from build123d import *

# Parameters (mm, degrees)
F1_DEPTH = 3


with BuildPart() as f1:
    # F0 (on Top) → F1 (new body)
    with BuildSketch(Plane.XY):
        with BuildLine():
            Line((16.723475, 5.431714), (8.751905, 14.74098))
            Line((8.751905, 14.74098), (4.802136, 11.358773))
            Line((4.802136, 11.358773), (-4.802136, 11.358773))
            Line((-4.802136, 11.358773), (-8.751905, 14.740979))
            Line((-8.751905, 14.740979), (-16.723475, 5.431713))
            Line((-16.723475, 5.431713), (-16.723475, 0))
            Line((-16.723475, 0), (-16.723475, -5.431713))
            Line((-16.723475, -5.431713), (-8.751905, -14.740979))
            Line((-8.751905, -14.740979), (-3.890651, -10.578264))
            Line((-3.890651, -10.578264), (-9.43802, -4.1))
            Line((-9.43802, -4.1), (-8.712763, -4.1))
            Line((-8.712763, -4.1), (-5.826839, -5.033681))
            ThreePointArc((-5.826839, -5.033681), (-4.72977, -6.076123), (-3.45, -6.883858))
            Line((-3.45, -6.883858), (-3.45, -14.2))
            Line((-3.45, -14.2), (3.45, -14.2))
            Line((3.45, -14.2), (3.45, -6.883857))
            ThreePointArc((3.45, -6.883857), (4.72977, -6.076123), (5.826838, -5.033681))
            Line((5.826838, -5.033681), (8.712763, -4.099999))
            Line((8.712763, -4.099999), (9.43802, -4.099999))
            Line((9.43802, -4.099999), (3.890651, -10.578264))
            Line((3.890651, -10.578264), (8.751905, -14.74098))
            Line((8.751905, -14.74098), (16.723475, -5.431714))
            Line((16.723475, -5.431714), (16.723475, 0))
            Line((16.723475, 0), (16.723475, 5.431714))
        make_face()
        with BuildLine():
            ThreePointArc((-2.25, -6.098155), (-3.833093, -5.249514), (-5.123475, -4))
            Line((-5.123475, -4), (-8.523475, -2.9))
            Line((-8.523475, -2.9), (-10.323475, -2.9))
            Line((-10.323475, -2.9), (-10.323475, -4))
            Line((-10.323475, -4), (-10.723475, -4))
            Line((-10.723475, -4), (-10.723475, -4.443783))
            Line((-10.723475, -4.443783), (-5.582645, -10.447288))
            Line((-5.582645, -10.447288), (-8.620929, -13.048985))
            Line((-8.620929, -13.048985), (-15.523475, -4.988134))
            Line((-15.523475, -4.988134), (-15.523475, 0))
            Line((-15.523475, 0), (-15.523475, 4.988134))
            Line((-15.523475, 4.988134), (-8.620929, 13.048985))
            Line((-8.620929, 13.048985), (-5.582645, 10.447288))
            Line((-5.582645, 10.447288), (-10.723475, 4.443783))
            Line((-10.723475, 4.443783), (-10.723475, 4))
            Line((-10.723475, 4), (-10.323475, 4))
            Line((-10.323475, 4), (-10.323475, 2.9))
            Line((-10.323475, 2.9), (-8.523475, 2.9))
            Line((-8.523475, 2.9), (-5.123475, 4))
            ThreePointArc((-5.123475, 4), (-3.028916, 5.751145), (-0.4, 6.487681))
            Line((-0.4, 6.487681), (-0.4, 7.3))
            Line((-0.4, 7.3), (0, 7.3))
            Line((0, 7.3), (0.4, 7.3))
            Line((0.4, 7.3), (0.4, 6.487681))
            ThreePointArc((0.4, 6.487681), (3.028916, 5.751145), (5.123475, 4))
            Line((5.123475, 4), (8.523475, 2.9))
            Line((8.523475, 2.9), (10.323475, 2.9))
            Line((10.323475, 2.9), (10.323475, 4))
            Line((10.323475, 4), (10.723475, 4))
            Line((10.723475, 4), (10.723475, 4.443783))
            Line((10.723475, 4.443783), (5.582645, 10.447288))
            Line((5.582645, 10.447288), (8.620929, 13.048985))
            Line((8.620929, 13.048985), (15.523475, 4.988134))
            Line((15.523475, 4.988134), (15.523475, 0))
            Line((15.523475, 0), (15.523475, -4.988134))
            Line((15.523475, -4.988134), (8.620929, -13.048985))
            Line((8.620929, -13.048985), (5.582645, -10.447288))
            Line((5.582645, -10.447288), (10.723475, -4.443783))
            Line((10.723475, -4.443783), (10.723475, -4))
            Line((10.723475, -4), (10.323475, -4))
            Line((10.323475, -4), (10.323475, -2.9))
            Line((10.323475, -2.9), (8.523475, -2.9))
            Line((8.523475, -2.9), (5.123475, -4))
            ThreePointArc((5.123475, -4), (3.833093, -5.249514), (2.25, -6.098155))
            Line((2.25, -6.098155), (2.25, -13))
            Line((2.25, -13), (-2.25, -13))
            Line((-2.25, -13), (-2.25, -6.098155))
        make_face(mode=Mode.SUBTRACT)
    extrude(amount=F1_DEPTH)


solid = f1.part
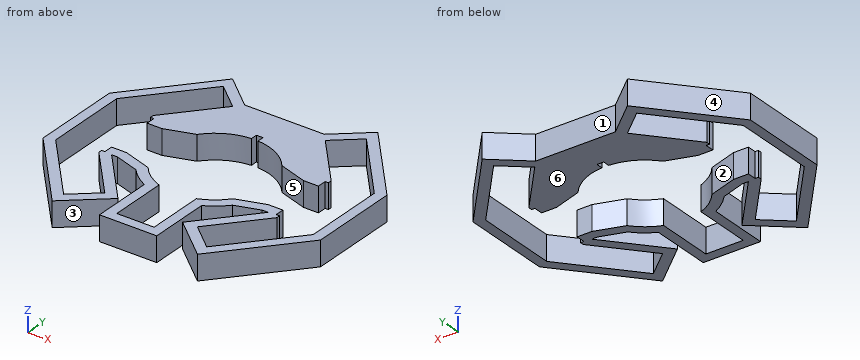
Input: part model. Units: mm. Frame: model coordinates. Face numbers are marked on the shaded views. A direction names the side the tool comes from. Coordinates: 2 decimals unless noted, no trailing zeros. Order: outer loops, then holes, each group sorted by start corner. A loop starts at its lowest first (then second) coordinate and runs counter-clockwise, first axis right, second up.
1. Contact query for flat-ended pins moving along their axis: P1, Ø1.4, axis at x = 9.5, z = 1, coming from the +Y side; P2, Ø1.5, axis at x = 0.5, z = 1, coming from the +Y side; P3, Ø1, axis at y = 7.5, z = 1.5, coming from the -X side. Output: stop coordinate, or through.
Checked values:
P1: stops at y = 14.68
P2: stops at y = 11.36
P3: stops at x = -15.38
2. Cut plane C-C, the plane y = 0.5. Return loops of the section in (x, z), plus the area to 3 significant figures.
Checked values:
outline: (-16.72, 0) - (-15.52, 0) - (-15.52, 3) - (-16.72, 3) - close; (15.52, 0) - (16.72, 0) - (16.72, 3) - (15.52, 3) - close
area: 7.20 mm2
3. Cut plane D-D, the plane y = -11. Return loops of the section in (x, z), plus the area to 3 significant figures.
Checked values:
outline: (-11.96, 0) - (-10.38, 0) - (-10.38, 3) - (-11.96, 3) - close; (-6.23, 0) - (-4.38, 0) - (-4.38, 3) - (-6.23, 3) - close; (-3.45, 0) - (-2.25, 0) - (-2.25, 3) - (-3.45, 3) - close; (2.25, 0) - (3.45, 0) - (3.45, 3) - (2.25, 3) - close; (4.38, 0) - (6.23, 0) - (6.23, 3) - (4.38, 3) - close; (10.38, 0) - (11.96, 0) - (11.96, 3) - (10.38, 3) - close
area: 27.7 mm2
4. Cut plane A-A, the plane y = -3.5. Return loops of the section in (x, z), plus the area to 3 significant figures.
Checked values:
outline: (-16.72, 0) - (-15.52, 0) - (-15.52, 3) - (-16.72, 3) - close; (-10.32, 0) - (-6.67, 0) - (-6.67, 3) - (-10.32, 3) - close; (6.67, 0) - (10.32, 0) - (10.32, 3) - (6.67, 3) - close; (15.52, 0) - (16.72, 0) - (16.72, 3) - (15.52, 3) - close
area: 29.1 mm2
5. Cut plane B-B, the plane x = -6.5. Return loops of the section in (y, z).
Checked values:
outline: (-12.81, 0) - (-11.23, 0) - (-11.23, 3) - (-12.81, 3) - close; (-9.38, 0) - (-7.53, 0) - (-7.53, 3) - (-9.38, 3) - close; (-4.82, 0) - (-3.55, 0) - (-3.55, 3) - (-4.82, 3) - close; (3.55, 0) - (9.38, 0) - (9.38, 3) - (3.55, 3) - close; (11.23, 0) - (12.81, 0) - (12.81, 3) - (11.23, 3) - close
6. Ray query, line 1 along Y through (x, z) = (4, 2.55); line 2 along X through (y, z) = (-1.75, 1.55); line 3 along X through (y, z) = (7, 0.75). Return the intervals inside material, ascending.
Checked values:
line 1: y = -10.67 to -10.45, -6.58 to -5.12, 5.12 to 11.36
line 2: x = -16.72 to -15.52, 15.52 to 16.72
line 3: x = -15.38 to -13.8, -8.53 to -0.4, 0.4 to 8.53, 13.8 to 15.38
7. Draft query along X for the marked faces 4, 5 and 6. Return one class per face: +X half, -X half, draft (parallel to the pull), parting line (faces both ways), or undercut.
Checked values:
face 4: -X half
face 5: undercut
face 6: draft
8. Access query for the marked faces 1, 2 and 3. Directions: +Z, -Z, +X, -X, +Y, -Y. A direction counts if a zero-diameter tool reaches every point of the face in a straight line with its end or side. Return the directions, or none.
Checked values:
face 1: +Z, -Z, +Y
face 2: +Z, -Z
face 3: +Z, -Z, -Y
